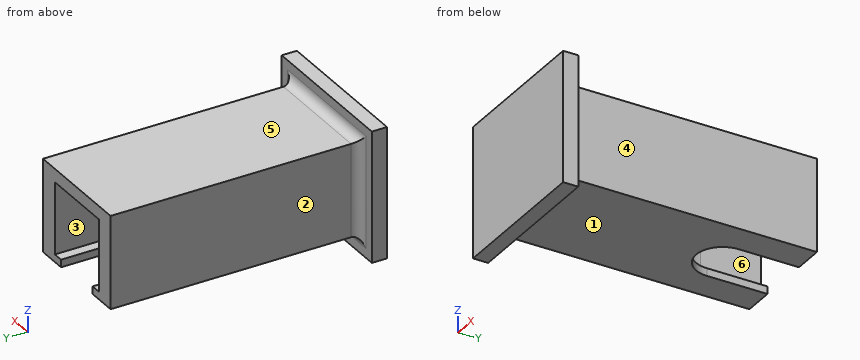
from build123d import *

# Parameters (mm, degrees)
BOSS_EXTRUDE1_DEPTH = 38
SKETCH3_W           = 60
SKETCH3_H           = 140
BOSS_EXTRUDE2_DEPTH = 7
BOSS_EXTRUDE3_DEPTH = 4
SKETCH5_W           = 80
SKETCH5_H           = 69
BOSS_EXTRUDE4_DEPTH = 8
FILLET1_R           = 5


with BuildPart() as part:
    # Sketch2 → Boss-Extrude1 (new body)
    with BuildSketch(Plane.XY):
        with BuildLine():
            Line((10.5, 108), (10.5, 140))
            Line((10.5, 140), (0, 140))
            Line((0, 140), (0, 0))
            Line((0, 0), (60, 0))
            Line((60, 0), (60, 140))
            Line((60, 140), (49.5, 140))
            Line((49.5, 140), (49.5, 108))
            ThreePointArc((49.5, 108), (30, 88.5), (10.5, 108))
        make_face()
    extrude(amount=BOSS_EXTRUDE1_DEPTH)

    # Sketch3 → Boss-Extrude2 (add)
    with BuildSketch(Plane.XY.offset(38)):
        with Locations((30, 70)):
            Rectangle(SKETCH3_W, SKETCH3_H)
    extrude(amount=BOSS_EXTRUDE2_DEPTH)

    # Sketch4 → Boss-Extrude3 (add)
    with BuildSketch(Plane(origin=(0, 0, 0), x_dir=(-1, 0, 0), z_dir=(0, 0, -1))):
        with BuildLine():
            Line((-44, 108), (-44, 140))
            Line((-44, 140), (-60, 140))
            Line((-60, 140), (-60, 0))
            Line((-60, 0), (0, 0))
            Line((0, 0), (0, 140))
            Line((0, 140), (-16, 140))
            Line((-16, 140), (-16, 108))
            ThreePointArc((-16, 108), (-30, 94), (-44, 108))
        make_face()
    extrude(amount=BOSS_EXTRUDE3_DEPTH)

    # Sketch5 → Boss-Extrude4 (add)
    with BuildSketch(Plane.XZ):
        with Locations((30, 20.5)):
            Rectangle(SKETCH5_W, SKETCH5_H)
    extrude(amount=-BOSS_EXTRUDE4_DEPTH)

    # Fillet1
    fillet1_edges = [part.edges().sort_by_distance(p)[0] for p in [
        (30, 8, -4),
        (30, 8, 45),
        (0, 8, 20.5),
        (60, 8, 20.5),
    ]]
    fillet(fillet1_edges, radius=FILLET1_R)


solid = part.part
Part model, mm, in its own coordinate system. Face numbers are marked on the shaded views. A direction names the side the tool comes from. Give positions to 0.01 mm unless a question says otherwise; leave off trailing zeros. Loops run counter-clockwise (first coordinate to the right, second up) from the corner with the lowest first, then second, coordinate; pieces in that order, holes last. Notation, with made-up numbers: (-4, 12) -> (38, 12) arc R15 cw to (38, 32) -> close; hole circle Ø6 at (-15.75, -18). An arc over 180 degrees is marked (long way). Write each question's results on one line, items separated by ' | '. Start each with the question number.
Q1. Pull direction Z, two halves, no side cores. Call the marked faces 4, 5 and 6: +Z half, -Z half, draft (parallel to the pull), parting line (faces both ways), or undercut.
Q2. Band-saw the part on B-B on y = 130. List the corners of the cut face in (x, z), plus the area to 3 significant figures.
Q3. Which spindle directions (+Z, -Z, +X, -X, +Y, -Y) get a long thin tool onto all of the face, cutting with end or side? Do the marked faces 1, 2 and 3. Say none if no direction does.
Q4. Band-saw the part on A-A on x = 57.5. List the corners of the cut face in (y, z), plus the area to 3 significant figures.
Q5. Band-saw the part on C-C on z = 41.5. List the corners of the cut face in (x, y).
Q6. Pin check, flat tips, straight feed: P1, Ø5, axis at x = 48, y = 88.5, coming from the -Z side; P2, Ø14.5, axis at y = 67.5, z = 8.5, coming from the +X side; P3, Ø9.5, axis at y = 131.5, z = 19, coming from the -X side. Stop position of each tip, or through.
Q7. Band-saw the part on D-D on x = 30. List the corners of the cut face in (y, z), plus the area to 3 significant figures.
Q8. Wall check: L1, parallel to Z at x = 57, y = 22; L2, parallel to X at y = 75.5, z = 37; L3, parallel to X at y = 129, z = 6. Give the ranges that are in metal, low to high.
Results are:
1) face 4: draft | face 5: +Z half | face 6: undercut
2) outline: (0, -4) -> (16, -4) -> (16, 0) -> (10.5, 0) -> (10.5, 38) -> (49.5, 38) -> (49.5, 0) -> (44, 0) -> (44, -4) -> (60, -4) -> (60, 45) -> (0, 45) -> close | area: 1,350 mm²
3) face 1: -Z, +X, -X, +Y | face 2: +Z, -Z, -X, +Y | face 3: +Y
4) outline: (0, -14) -> (8, -14) -> (8, -9) arc R5 cw to (13, -4) -> (140, -4) -> (140, 45) -> (13, 45) arc R5 cw to (8, 50) -> (8, 55) -> (0, 55) -> close | area: 7,030 mm²
5) outline: (-10, 0) -> (70, 0) -> (70, 8) -> (65, 8) arc R5 cw to (60, 13) -> (60, 140) -> (0, 140) -> (0, 13) arc R5 cw to (-5, 8) -> (-10, 8) -> close
6) P1: stops at z = -4 | P2: stops at x = 60 | P3: stops at x = 0
7) outline: (0, -14) -> (8, -14) -> (8, -9) arc R5 cw to (13, -4) -> (94, -4) -> (94, 0) -> (88.5, 0) -> (88.5, 38) -> (140, 38) -> (140, 45) -> (13, 45) arc R5 cw to (8, 50) -> (8, 55) -> (0, 55) -> close | area: 4,890 mm²
8) L1: z = -4 to 45 | L2: x = 0 to 60 | L3: x = 0 to 10.5, 49.5 to 60
